Could you check a few things on this drawing? It's one solid part, dimensions in mm from its lowest x, y, z. Coordinates: 2 decimals unless noted, no trailing zeros. Order: outer loops, then holes, each group sorted by start corner. A loop starts at its lowest first (then second) coordinate and runs counter-clockwise, first axis right, second up. Notation, with made-up numbers: M 30.25,19.25 L 79.25,19.25 A5 cw 79.25,24.25 Z; hole C -5.75,39 d1. An arc over 180 degrees is marked long. Write item = value, one per line. Start each with the question number.
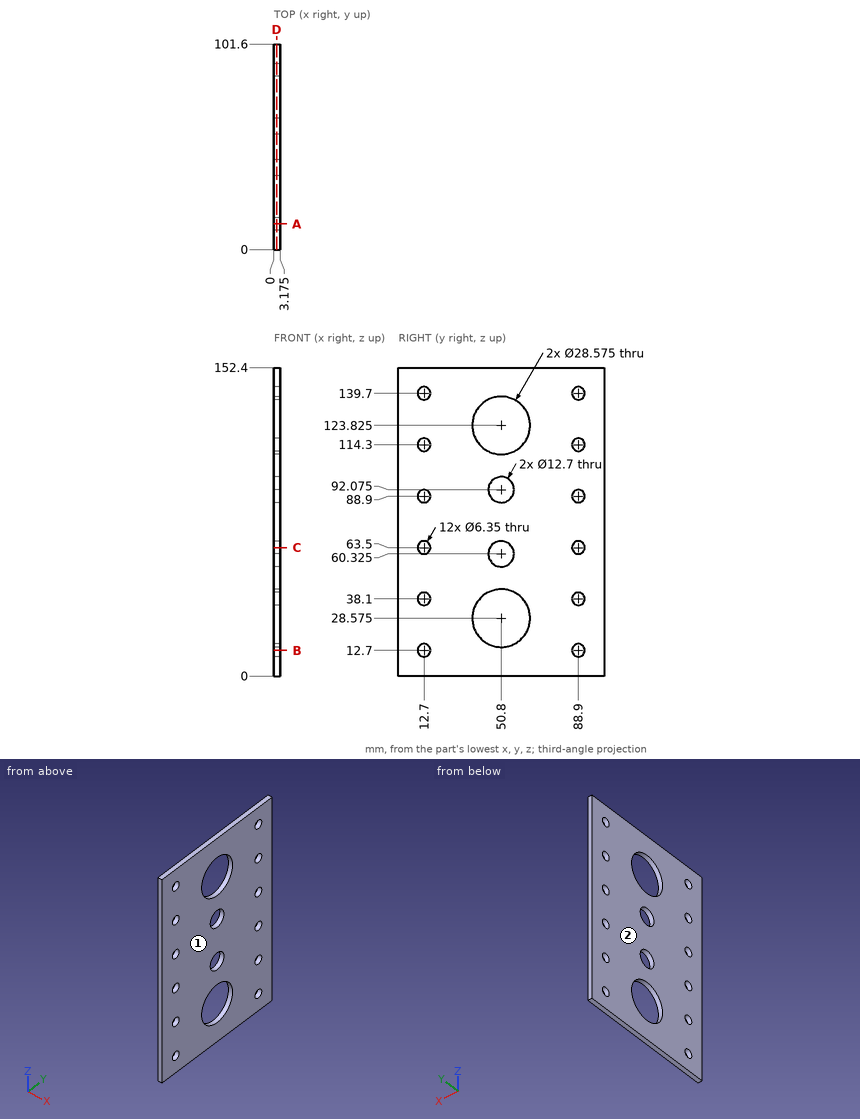
(1) Imagine slicing it at D-D on x = 1.3. Give the number of separate pieces and of enclosed holes in the cut face, plus the area to 3 significant figures.
(2) Thinking about a two-plate mould opening in X: for the marked faces 1 and 2, which applies, released by +X, released by -X, zero draft, split by the parting line, or undercut?
(3) Imagine slicing it at B-B on z = 12.7. List the corners of the cut face in (x, y) for me (3 decimals), plus the area to 3 significant figures.
(4) Imagine slicing it at A-A on y = 12.7. List the corners of the cut face in (x, z) for me (3 decimals).
(5) Please list where these lines run through material, in increasing order: probe 1 along Z at (x, y) = (0.7, 50.8) (1 decimal); probe 2 along Y at (x, z) = (2.1, 64.5); probe 3 along Y at (x, z) = (2.4, 61). Write a range as from..to.
(6) Will these pins go through, and if not, where does the flat tip stop? P1, Ø5, axis at y = 63, z = 117.5, coming from the +X side (3 decimals); P2, Ø17, axis at y = 50.8, z = 28.575, coming from the +X side.
(7) Imagine slicing it at C-C on z = 63.5. List the corners of the cut face in (x, y) for me (3 decimals), plus the area to 3 significant figures.
Response:
q1.separate_pieces = 1
q1.enclosed_holes = 16
q1.area = 13,600 mm2
q2.face_1 = released by +X
q2.face_2 = released by -X
q3.outline = M 0,0 L 3.175,0 L 3.175,9.525 L 0,9.525 Z; M 0,15.875 L 3.175,15.875 L 3.175,85.725 L 0,85.725 Z; M 0,92.075 L 3.175,92.075 L 3.175,101.6 L 0,101.6 Z
q3.area = 282 mm2
q4.outline = M 0,0 L 3.175,0 L 3.175,9.525 L 0,9.525 Z; M 0,15.875 L 3.175,15.875 L 3.175,34.925 L 0,34.925 Z; M 0,41.275 L 3.175,41.275 L 3.175,60.325 L 0,60.325 Z; M 0,66.675 L 3.175,66.675 L 3.175,85.725 L 0,85.725 Z; M 0,92.075 L 3.175,92.075 L 3.175,111.125 L 0,111.125 Z; M 0,117.475 L 3.175,117.475 L 3.175,136.525 L 0,136.525 Z; M 0,142.875 L 3.175,142.875 L 3.175,152.4 L 0,152.4 Z
q5.probe_1 = 0..14.3, 42.9..54, 66.7..85.7, 98.4..109.5, 138.1..152.4
q5.probe_2 = 0..9.69, 15.71..46.02, 55.58..85.89, 91.91..101.6
q5.probe_3 = 0..10.74, 14.66..44.49, 57.11..86.94, 90.86..101.6
q6.P1 = 3.175
q6.P2 = through
q7.outline = M 0,0 L 3.175,0 L 3.175,9.525 L 0,9.525 Z; M 0,15.875 L 3.175,15.875 L 3.175,45.301 L 0,45.301 Z; M 0,56.299 L 3.175,56.299 L 3.175,85.725 L 0,85.725 Z; M 0,92.075 L 3.175,92.075 L 3.175,101.6 L 0,101.6 Z
q7.area = 247 mm2
